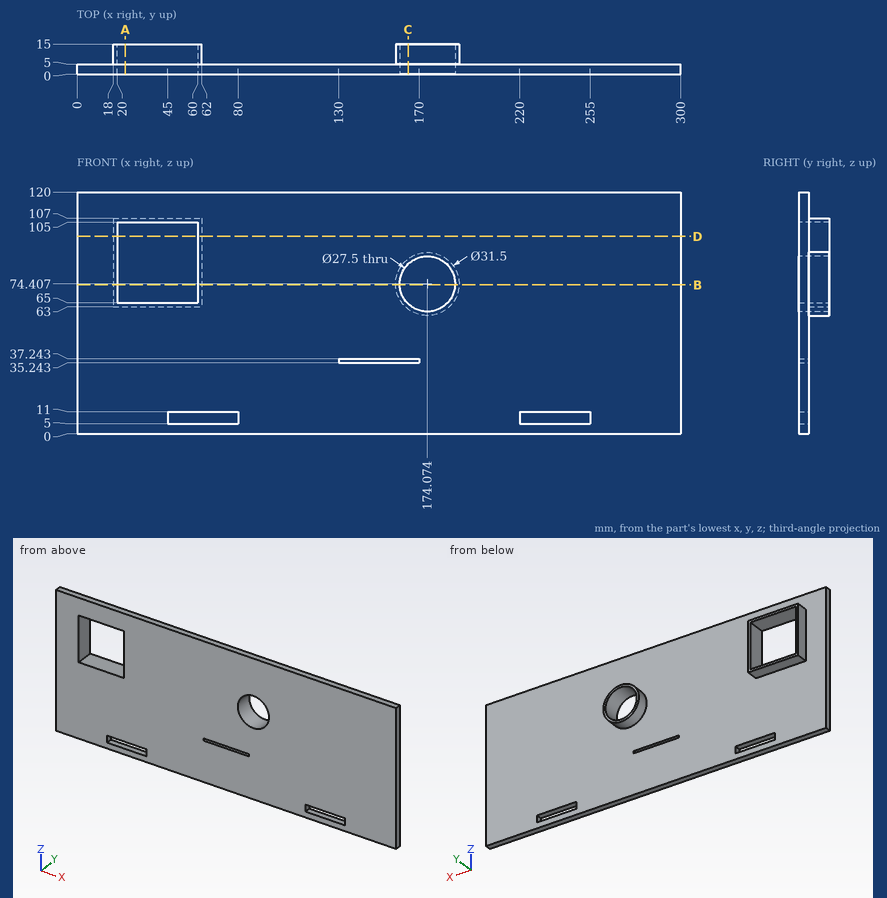
Can you work these out from the drawing? Everything is in mm from the part's minimum corner. Coordinates: 2 decimals unless noted, no trailing zeros. Loops run counter-clockwise (first coordinate to the right, second up) from the corner with the lowest first, then second, coordinate; pieces in that order, holes last. Notation, with made-up numbers: (-13.75, 80) -> (12.25, 80) arc R10 ccw to (12.25, 97) -> close; hole circle Ø8 at (76.5, 84.5). An arc over 180 degrees is marked (long way). Return JSON: item names as keys, results as strings.
1) If we section it at C-C, the plane x = 164.5: Write out the boundary of the cut face in (y, z).
Results below:
{"outline": "(0, 0) -> (5, 0) -> (5, 35.24) -> (0, 35.24) -> close; (0, 37.24) -> (5, 37.24) -> (5, 61.9) -> (15, 61.9) -> (15, 64.54) -> (0, 64.54) -> close; (0, 84.28) -> (15, 84.28) -> (15, 86.91) -> (5, 86.91) -> (5, 120) -> (0, 120) -> close"}
2) If we section it at B-B, the plane z = 74: Write out the boundary of the cut face in (x, y), then the cut area to 3 significant figures.
Results below:
{"outline": "(0, 0) -> (20, 0) -> (20, 15) -> (18, 15) -> (18, 5) -> (0, 5) -> close; (60, 0) -> (160.33, 0) -> (160.33, 15) -> (158.33, 15) -> (158.33, 5) -> (62, 5) -> (62, 15) -> (60, 15) -> close; (187.82, 0) -> (300, 0) -> (300, 5) -> (189.82, 5) -> (189.82, 15) -> (187.82, 15) -> close", "area": "1,240 mm²"}
3) If we section it at A-A, the plane x = 24: Write out the boundary of the cut face in (y, z).
Results below:
{"outline": "(0, 0) -> (5, 0) -> (5, 63) -> (15, 63) -> (15, 65) -> (0, 65) -> close; (0, 105) -> (15, 105) -> (15, 107) -> (5, 107) -> (5, 120) -> (0, 120) -> close"}
4) I need wall thicknesses on line 1 (X direction, y = 2.5, z = 73.5) (1 decimal); line 2 (X direction, y = 4.25, z = 10); line 3 (Z direction, x = 66, y = 1.5). Which ranges of each line are inside material? Lowest first, please. Write a range as from..to.
Results below:
{"line 1": "0..20, 60..160.4, 187.8..300", "line 2": "0..45, 80..220, 255..300", "line 3": "0..5, 11..120"}
5) Will these pins go through, and if not, where does the flat tip stop? pin 1 (4.5 mm diameter, centred on x = 36, y = 10.5, fed in from -Z); pin 2 (8 mm diameter, centred on y = 9.5, z = 89, fed in from -X); pin 3 (5 mm diameter, centred on x = 60, z = 47.5, fed in from +Y).
Results below:
{"pin 1": "z = 63", "pin 2": "x = 18", "pin 3": "y = 5"}
6) If we section it at D-D, the plane z = 98: Write out the boundary of the cut face in (x, y), then the cut area to 3 significant figures.
Results below:
{"outline": "(0, 0) -> (20, 0) -> (20, 15) -> (18, 15) -> (18, 5) -> (0, 5) -> close; (60, 0) -> (300, 0) -> (300, 5) -> (62, 5) -> (62, 15) -> (60, 15) -> close", "area": "1,340 mm²"}
